Here's how the part is built. I have some questions about the finished solid (model axes, mm). A direction names the side the tool comes from. Give positions to 0.01 mm unless a question says otherwise; leave off trailing zeros. Loops run counter-clockwise (first coordinate to the right, second up) from the corner with the lowest first, then second, coordinate; pieces in that order, holes last. Notation, with made-up numbers: (-29.75, -20.75) - (-21.75, -20.75) arc R29 cw to (-21.75, 17.25) - close; hole circle Ø4 at (-15, 61). An arc over 180 degrees is marked (long way). Use a Markdown table: item, result.
from build123d import *

# Parameters (mm, degrees)
PAD_DEPTH         = 1
PAD004_DEPTH      = 20
FILLET_R          = 10
FILLET001_R       = 2
PAD005_DEPTH      = 35
PAD005_DEPTH_BACK = 1
SKETCH005_R       = 9.6
POCKET_DEPTH      = 86.945705044


with BuildPart() as part:
    # Sketch → Pad (new body)
    with BuildSketch(Plane.XY):
        with BuildLine():
            ThreePointArc((2.407e-07, 65), (-39.2503215588, 51.8113139915), (-62.5726380514, 17.5973))
            ThreePointArc((-62.5726380514, 17.5973), (-62.2816568518, 16.2569186959), (-61.1956, 15.4192))
            Line((-61.1956, 15.4192), (-48.0942, 15.4192))
            ThreePointArc((-48.0942, 15.4192), (-46.0175682638, 16.2684180018), (-44.5213344809, 17.9402))
            ThreePointArc((44.6290648541, 17.6705), (0.1452101265, 47.9997803539), (-44.5213344809, 17.9402))
            ThreePointArc((44.6290648541, 17.6705), (45.6957884662, 16.2979684833), (47.1679586113, 15.3736))
            Line((47.1679586113, 15.3736), (54.9232114248, 15.3841578001))
            ThreePointArc((54.9232114248, 15.3841578001), (76.1100083043, 24.1853710213), (84.8823702407, 45.38413))
            Line((84.8823702407, 59.61183), (84.8823702407, 45.38413))
            ThreePointArc((84.8823702407, 59.61183), (83.3042117859, 63.4218415452), (79.4942002407, 65))
            Line((2.407e-07, 65), (79.4942002407, 65))
        make_face()
    extrude(amount=PAD_DEPTH)

    # Sketch001 → Pad004 (new body)
    with BuildSketch(Plane.XY.offset(1)):
        with BuildLine():
            ThreePointArc((6.04881e-05, 65), (-39.6936405321, 51.4724674103), (-62.8655421025, 16.5204))
            Line((-62.8655421025, 16.5204), (-59.7655421025, 16.5204))
            ThreePointArc((6.04881e-05, 63), (-37.8013201978, 49.9422727575), (-59.7655421025, 16.5204))
            Line((80.0000604881, 63), (6.04881e-05, 63))
            Line((80.0000604881, 65), (80.0000604881, 63))
            Line((6.04881e-05, 65), (80.0000604881, 65))
        make_face()
    extrude(amount=PAD004_DEPTH)

    # Fillet
    fillet_edges = [part.edges().sort_by_distance(p)[0] for p in [
        (80.00006, 64, 21),
    ]]
    fillet(fillet_edges, radius=FILLET_R)

    # Fillet001
    fillet001_edges = [part.edges().sort_by_distance(p)[0] for p in [
        (-61.315542, 16.5204, 21),
    ]]
    fillet(fillet001_edges, radius=FILLET001_R)

    # Sketch004 → Pad005 (new body, two sides)
    with BuildSketch(Plane.XY.offset(1)) as pad005_sk:
        Polygon((12.8190404688, 80.7158918092), (41.0807640524, 70.6523447167), (39.0680546339, 65), (7.2228631212, 65), align=None)
    extrude(amount=PAD005_DEPTH)
    extrude(pad005_sk.sketch, amount=-PAD005_DEPTH_BACK)

    # Sketch005 → Pocket (cut, through all)
    with BuildSketch(Plane(origin=(26.9499022606, 75.6841182629, 0), x_dir=(-0.9420574528, 0.3354515698, 0), z_dir=(0.3354515698, 0.9420574528, 0))):
        with Locations((0, 35)):
            Circle(SKETCH005_R)
    extrude(amount=-POCKET_DEPTH, mode=Mode.SUBTRACT)


solid = part.part
(1) Suppose I cut it at D-D on z = 27. Write out the boundary of the cut face in (x, y).
A:
| item | result |
|---|---|
| outline | (7.22, 65) - (17.51, 65) - (21.95, 77.46) - (12.82, 80.72) - close; (28.78, 65) - (39.07, 65) - (41.08, 70.65) - (31.95, 73.9) - close |
(2) On a 3-axis mill with a long thin cutter (end or side, diameter ignored), from which of +Z, -Z, +X, -X, +Y, -Y can I reach the whole of each face in a straight line? I mean faces 1 (the face through (41, 63, 11)), 2 (the face through (-61, 16.52, 10)), 3 (the face through (4, 65, 10)). Say none if no direction works.
A:
| item | result |
|---|---|
| face 1 | +Z, +X, -Y |
| face 2 | +Z, +X, -X, -Y |
| face 3 | +Z, -Z, -X, +Y |
(3) If I drill on line 1 (Z direction, x = 19, y = 61.5); line 2 (Y direction, x = 48.5, z = 6); line 3 (X direction, y = 70.5, z = 27.5) (3 decimals), over which ranges is the centre line in solid material (lowest first)?
A:
| item | result |
|---|---|
| line 1 | 0 to 1 |
| line 2 | 63 to 65 |
| line 3 | 9.181 to 18.743, 31.465 to 41.027 |
(4) Suppose I cut it at A-A on z = 9. Write out the boundary of the cut face in (x, y), plus the area to 3 significant figures.
A:
| item | result |
|---|---|
| outline | (-62.87, 16.52) - (-59.77, 16.52) arc R62 cw to (0, 63) - (80, 63) - (80, 65) - (39.07, 65) - (41.08, 70.65) - (12.82, 80.72) - (7.22, 65) - (0, 65) arc R65 ccw to start |
| area | 702 mm2 |
(5) Suppose I cut it at B-B on y = 31.5. Write out the boundary of the cut face in (x, z), plus the area to 3 significant figures.
A:
| item | result |
|---|---|
| outline | (-56.86, 0) - (-36.22, 0) - (-36.22, 1) - (-53.72, 1) - (-53.72, 21) - (-56.86, 21) - close; (36.22, 0) - (81.48, 0) - (81.48, 1) - (36.22, 1) - close |
| area | 129 mm2 |
(6) Suppose I cut it at C-C on x = 37.5. Write out the boundary of the cut face in (y, z), plus the area to 3 significant figures.
A:
| item | result |
|---|---|
| outline | (29.96, 0) - (71.93, 0) - (71.93, 36) - (65, 36) - (65, 21) - (63, 21) - (63, 1) - (29.96, 1) - close |
| area | 324 mm2 |
(7) Will these pins go through, and if not, where does the flat tip stop? pin 1 (2 mm diameter, centred on y = 63.5, z = 4, fed in from +X); pin 2 (6 mm diameter, centred on y = 46, z = 16, fed in from +X); pin 3 (6 mm diameter, centred on x = 0.5, z = 12, fed in from -Y).
A:
| item | result |
|---|---|
| pin 1 | x = 80 |
| pin 2 | x = -38.98 |
| pin 3 | y = 62.94 |
(8) We'd pull the mould along Y, two halves only. Please class faces 4 (the face through (40.1, 67.9, 18.3)), 5 (the face through (27, 46, 1)), 6 (the face through (0.95, 47.99, 0.49)): pulls with the +Y half, pulls with the -Y half, needs draft (parallel to the pull), parting line crosses it, or undercut.
A:
| item | result |
|---|---|
| face 4 | undercut |
| face 5 | needs draft |
| face 6 | pulls with the -Y half |
